The listing builds one solid part. Answer for the finished solid, in the listing's coordinates (mm). A direction names the side the tool comes from. Coordinates: 2 decimals unless noted, no trailing zeros. Loops run counter-clockwise (first coordinate to the right, second up) from the corner with the lowest first, then second, coordinate; pieces in that order, holes last. Notation, with made-up numbers: (48.5, 62.5) - (106.5, 62.5) arc R13 ccw to (106.5, 85.5) - close; hole circle Ø4 at (-4.75, 8). An arc over 180 degrees is marked (long way). Put each result on its own line as item: value.
```python
from build123d import *

# Parameters (mm, degrees)
F0_W     = 914.4
F0_H     = 914.4
F1_DEPTH = 1219.2
F2_R     = 112.2615
F2_R_2   = 94.92904
F2_R_3   = 152.671278
F2_R_4   = 148.211115
F3_DEPTH = 30.48
F4_W     = 646.188111
F4_H     = 106.785357
F5_DEPTH = 30.48


with BuildPart() as f1:
    # F0 (on Top) → F1 (new body)
    with BuildSketch(Plane.XY):
        with Locations((4.408748, 9.645843)):
            Rectangle(F0_W, F0_H)
    extrude(amount=F1_DEPTH)

    # F2 (on face) → F3 (join)
    with BuildSketch(Plane.XY.offset(1219.2)):
        with Locations((-263.714761, 314.844251)):
            Circle(F2_R)
        with Locations((294.854611, -298.486859)):
            Circle(F2_R_2)
        with Locations((182.593152, 172.46379)):
            Circle(F2_R_3)
        with Locations((-181.572214, -167.058766)):
            Circle(F2_R_4)
    extrude(amount=F3_DEPTH)

    # F4 (on face) → F5 (join)
    with BuildSketch(Plane.XZ.offset(447.554157)):
        with Locations((10.093763, 991.878598)):
            Rectangle(F4_W, F4_H)
    extrude(amount=F5_DEPTH)


solid = f1.part
```
1) The part is cut by section D-D (y = -412). Give the vertices of the cut face in (x, z).
Found:
outline: (-452.79, 0) - (461.61, 0) - (461.61, 1219.2) - (-452.79, 1219.2) - close
2) The part is cut by section B-B (y = -144). Give the vertices of the cut face in (x, z), and give its area (3 significant figures).
Found:
outline: (-452.79, 0) - (461.61, 0) - (461.61, 1219.2) - (-35.17, 1219.2) - (-35.17, 1249.68) - (-327.98, 1249.68) - (-327.98, 1219.2) - (-452.79, 1219.2) - close
area: 1,120,000 mm^2
3) For a pull along Y with two mould halves and no side action, classify faces 1 (the face through (-184, -165, 1249.68)), 2 (the face through (-160.014, 271.847, 1234.227)), 3 (the face through (6, -478.034, 993)) as pulls with the +Y half, pulls with the -Y half, needs draft (parallel to the pull), parting line crosses it, or undercut.
Found:
face 1: needs draft
face 2: undercut
face 3: pulls with the -Y half
4) The part is cut by section A-A (x = -102.5). Give the vertices of the cut face in (y, z), and give its area (3 significant figures).
Found:
outline: (-478.03, 938.49) - (-447.55, 938.49) - (-447.55, 0) - (466.85, 0) - (466.85, 1219.2) - (-41.7, 1219.2) - (-41.7, 1249.68) - (-292.41, 1249.68) - (-292.41, 1219.2) - (-447.55, 1219.2) - (-447.55, 1045.27) - (-478.03, 1045.27) - close
area: 1,130,000 mm^2
5) For faces 4 (the face through (6, -463, 938.486)), 5 (the face through (224.89, -234.33, 1234.23)), 6 (the face through (6, -463, 1045.271)), 7 (the face through (-313, -463, 991)), determine the directions among +Z, -Z, +X, -X, +Y, -Y from which every point of the face is accessible in a straight line to the end or side of a thin tool.
Found:
face 4: -Z, +X, -X, -Y
face 5: +Z
face 6: +Z, +X, -X, -Y
face 7: +Z, -Z, -X, -Y
6) The part is cut by section C-C (z = 817.5). Give the vertices of the cut face in (x, y), and give its area (3 significant figures).
Found:
outline: (-452.79, -447.55) - (461.61, -447.55) - (461.61, 466.85) - (-452.79, 466.85) - close
area: 836,000 mm^2
7) Each of these flat-tipped pins is pushed along its axis until it touches: pin 1 (1 mm diameter, centred on x = -81.5, z = 892, fed in from -Y); pin 2 (9 mm diameter, centred on y = -466.5, z = 978, fed in from -X); pin 3 (9 mm diameter, centred on x = -118, y = -470.5, fed in from -Z); pin 4 (4 mm diameter, centred on x = 156, y = -235.5, fed in from -Z). Where does it stop, or does it pass through?
Found:
pin 1: stops at y = -447.55
pin 2: stops at x = -313
pin 3: stops at z = 938.49
pin 4: stops at z = 0
8) Straight lines are drawn through the part: L1, parallel to Y at x = -368, z = 723.5; L2, parallel to Z at x = 335, y = -22. For each, find the intervals that lie inside material, in ascending order. Write a range as [from, to].
Found:
L1: y = [-447.55, 466.85]
L2: z = [0, 1219.2]
